Read the model definition and answer for the solid it produces. Units are mm, in the model's axes. Face numbers are marked on the shaded views. A direction names the side the tool comes from. Coordinates: 2 decimals unless noted, no trailing zeros. Write each loop counter-clockwise with the first axis right and the second up, starting at its lowest first coordinate (ties: lowest second). Pieces come first, ordered by that corner, then holes.
Item 1: Section D-D (y = 51) is taken. Give the vertices of the cut face in (x, z), then the cut area to 3 significant figures.
Item 2: Section C-C (x = 95) is taken. Give the vertices of the cut face in (y, z).
Item 3: Straight lines are drawn through the part: probe 1 along X at (y, z) = (66.95, 55); probe 2 along X at (y, z) = (80, 55); probe 3 along Z at (x, y) = (45, 79.5). For each, find the intervals that lie inside material, in ascending order.
Item 4: Section B-B (y = 68) is taken. Give the vertices of the cut face in (x, z).
Item 5: Section A-A (z = 55) is taken. Give the vertices of the cut face in (x, y).
Item 6: Determine the mould class of the marked faces 1, 2, 3 and 4 for opening direction X: released by +X, released by -X, zero draft, split by the parting line, or undercut.
Item 7: Each of these flat-tipped pins is pushed along its axis until it touches: P1, Ø8, axis at x = 109, z = 33.5, coming from the -Y side; P2, Ø5, axis at x = 83.5, z = 13.5, coming from the -Y side; P3, Ø1.5, axis at x = 87, y = 57, coming from the +Z side; P4, Ø13, axis at x = 97.5, z = 52.5, coming from the -Y side. Where does it stop, or does it pass through?
Item 8: A tool of negligible diameter and unlimited length cuts with its end or side. For the marked faces 5, 6 and 7, from which of +Z, -Z, +X, -X, +Y, -Y can it reach the whole face along a straight path? Write none if from no direction.
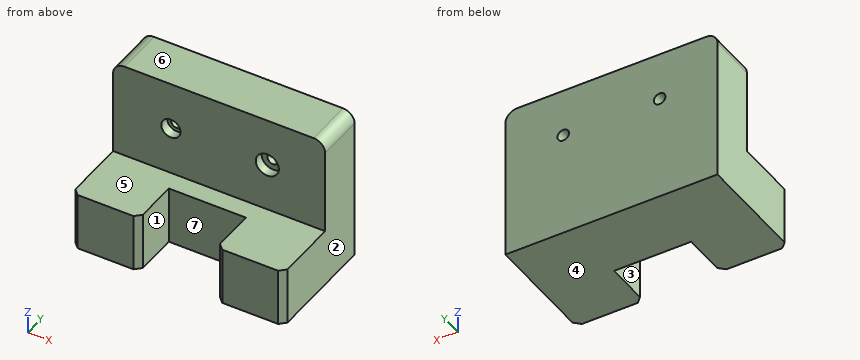
Autodesk Fusion 360 part; units mm, degrees
sketch "Sketch1" plane through (0, 0, 0) normal (0, 0, 1) x (1, 0, 0)
  line L0 (15, 30) -> (50, 30)
  line L1 (50, 30) -> (50, 55)
  line L2 (50, 55) -> (90, 55)
  line L3 (90, 55) -> (90, 30)
  line L4 (90, 30) -> (125, 30)
  line L5 (15, 30) -> (15, 90)
  line L6 (125, 30) -> (125, 90)
  line L7 (15, 90) -> (125, 90)
  dimension "d6" = 60
extrude "Extrude1" add sketch "Sketch1" along normal blind 30 makes body 1
chamfer "Chamfer1" distance 3 angle 45 1 edges at (50, 30, 15) on bodies 1
chamfer "Chamfer2" distance 3 angle 45 1 edges at (90, 30, 15) on bodies 1
chamfer "Chamfer3" distance 3 angle 45 1 edges at (125, 30, 15) on bodies 1
chamfer "Chamfer4" distance 3 angle 45 1 edges at (15, 30, 15) on bodies 1
sketch "Sketch2" plane through (0, 0, 0) normal (0, 0, 1) x (1, 0, 0)
  line L0 (15, 90) -> (15, 65)
  line L1 (15, 65) -> (125, 65)
  line L2 (125, 65) -> (125, 90)
  line L3 (125, 90) -> (15, 90)
extrude "Extrude2" add sketch "Sketch2" along normal blind 80 separate body makes body 2
combine "Combine1" operation add target body 1 tool bodies 2
fillet "Fillet1" radius 6 1 edges at (125, 77.5, 80) on bodies 1
fillet "Fillet2" radius 6 1 edges at (15, 77.5, 80) on bodies 1
sketch "Sketch3" plane through (0, 0, 0) normal (0, 1, 0) x (1, 0, 0)
hole "Hole1" at (45, 65, 55) direction (0, 1, 0) diameter 6 depth 25 tip angle 180 counterbore diameter 10 counterbore depth 5 bodies 1
hole "Hole2" at (95, 65, 55) direction (0, 1, 0) diameter 6 depth 25 tip angle 180 counterbore diameter 12 counterbore depth 5 bodies 1
Established:
1. outline: (15, 0) - (50, 0) - (50, 30) - (15, 30) - close; (90, 0) - (125, 0) - (125, 30) - (90, 30) - close
1. area: 2,100 mm2
2. outline: (30, 0) - (90, 0) - (90, 52) - (70, 52) - (70, 49) - (65, 49) - (65, 30) - (30, 30) - close; (65, 61) - (70, 61) - (70, 58) - (90, 58) - (90, 80) - (65, 80) - close
3. probe 1: x = 15 to 40, 50 to 89, 101 to 125
3. probe 2: x = 15 to 42, 48 to 92, 98 to 125
3. probe 3: z = 0 to 52, 58 to 80
4. outline: (15, 0) - (125, 0) - (125, 74) arc R6 ccw to (119, 80) - (21, 80) arc R6 ccw to (15, 74) - close; hole circle Ø10 at (45, 55); hole circle Ø12 at (95, 55)
5. outline: (15, 65) - (40, 65) - (40, 70) - (42, 70) - (42, 90) - (15, 90) - close; (48, 70) - (50, 70) - (50, 65) - (89, 65) - (89, 70) - (92, 70) - (92, 90) - (48, 90) - close; (98, 70) - (101, 70) - (101, 65) - (125, 65) - (125, 90) - (98, 90) - close
6. face 1: undercut
6. face 2: released by +X
6. face 3: undercut
6. face 4: zero draft
7. P1: stops at y = 30
7. P2: stops at y = 55
7. P3: stops at z = 30
7. P4: stops at y = 65
8. face 5: +Z, +X, -X, -Y
8. face 6: +Z, +X, -X, +Y, -Y
8. face 7: +Z, -Z, -Y
